Input: dimensioned drawing with shaded views. Units: mm. Origin: part minimum x, y, z. Round coordinates to 2 decimals unless told otherwise and drop trailing zeros. Loops run counter-clockwise (first coordinate to the right, second up) from the corner with the lowest first, then second, coordinate; pieces in that order, holes last. Notation, with made-up numbers: M 85,25 L 129,25 A12 cw 129,40 Z; hole C -29.5,-6 d11. An arc over 180 degrees is marked long. One line per item, written item: value.
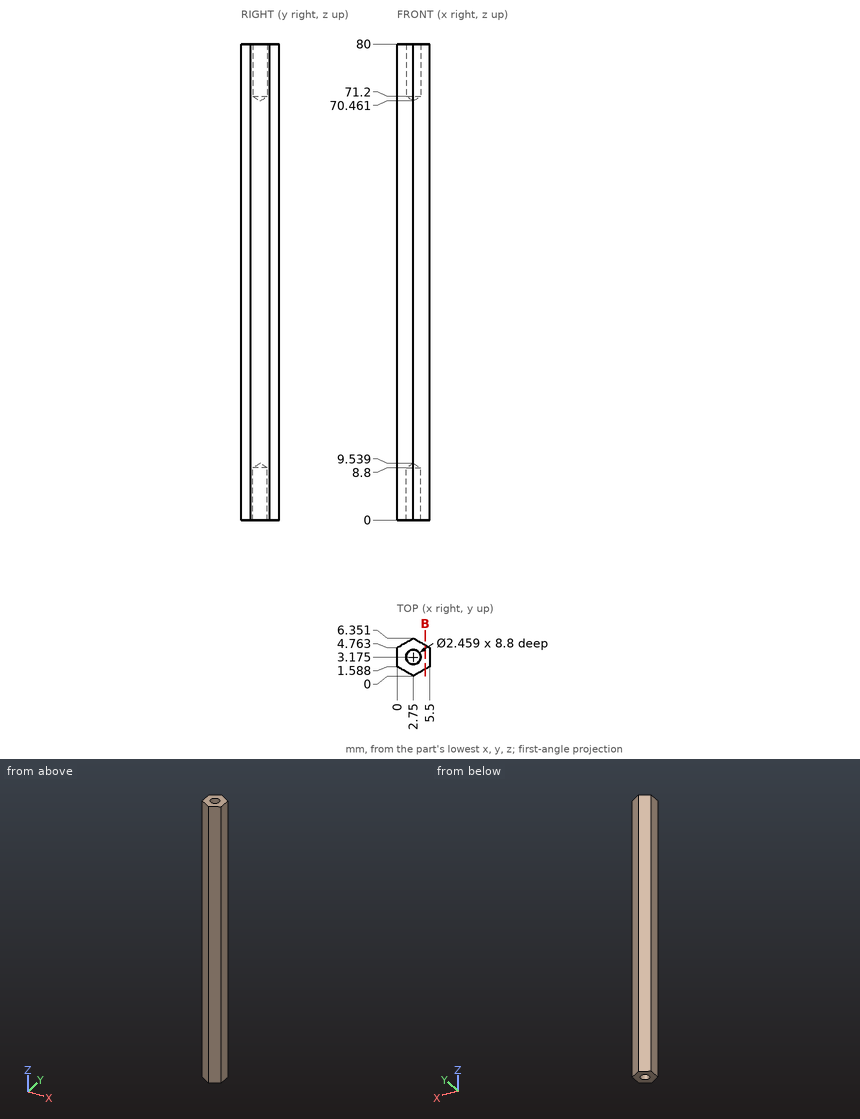
1. Ray query, line 1 (X direction, y = 3.25, z = 4); line 2 (Y direction, x = 1.2, z = 63) (1 decimal); line 3 (Y direction, x = 2.6, z = 38.5) (1 decimal). Return the intervals inside material, ascending. Write a range as [from, to].
Report:
line 1: x = [0, 1.52], [3.98, 5.5]
line 2: y = [0.9, 5.5]
line 3: y = [0.1, 6.3]
2. Section query B-B (x = 4.7). Return the cut outline in (y, z) (1 decimal).
Report:
outline: M 1.1,0 L 5.2,0 L 5.2,80 L 1.1,80 Z
3. Pin query (flat end, axial travel): pin 1 (2 mm diameter, centred on y = 4, z = 60, fed in from -X); pin 2 (1 mm diameter, centred on x = 1.5, z = 34.5, fed in from +Y). Return the tip coordinate at first contact, or that it passes through.
Report:
pin 1: stops at x = 0
pin 2: stops at y = 5.92
